Model file for the job. Use its own axes, mm. A direction names the side the tool comes from. Round coordinates to 2 decimals unless told otherwise and drop trailing zeros. Loops run counter-clockwise (first coordinate to the right, second up) from the corner with the lowest first, then second, coordinate; pieces in that order, holes last. Notation, with made-up numbers: M 66.5,35 L 107.5,35 A16 ccw 107.5,61 Z; hole C -13,-7 d8. An arc over 180 degrees is marked long. Use a Markdown table: item, result. Add a question column.
Q1. Cut at B-B (x = 0). Give the cut face in (y, z).
Q2. Cut at A-A (z = 7). Give the cut face in (x, y), plus the area to 3 significant figures.
Q3. Cut at C-C (y = -20). Give the cut face in (x, z).
Q4. Tool access for faces 1 (the face through (-17.062, -15.477, 6.873)), 2 (the face through (19.894, -30.203, 7.194)), 3 (the face through (-6, -20, 2)), 4 (the face through (-19.894, -30.203, 7.194)), 5 (the face through (17.062, -15.477, 6.873)): list every direction of +Z, -Z, +X, -X, +Y, -Y with a clear straight run to the whole face (end or side of a thin tool).
Q5. Probe line 1 (Y direction, x = 0, z = 5.6); line 2 (Y direction, x = 0, z = 1.75); line 3 (X direction, y = -20, z = 1.15). List the from-to ranges inside material, lowest first. Write a range as from..to.
Q6. Pin check, flat tips, straight feed: pin 1 (4 mm diameter, centred on y = -19, z = 4.5, fed in from -X); pin 2 (5 mm diameter, centred on x = 0, y = -20, fed in from +Z); pin 3 (1 mm diameter, centred on x = -5.5, z = 4, fed in from -Y); pin 4 (2 mm diameter, centred on y = -25, z = 4.5, fed in from -X). Stop position of each tip, or through.
Q7. Cut at D-D (x = -16). Give the cut face in (y, z), plus the area to 3 significant figures.
Q8. Mould opens along X. For faces 6 (the face through (3, -17, 4)), 7 (the face through (14.077, -0.376, 3.246)), 8 (the face through (0, 0, 4)), 9 (the face through (-20.23, -30.04, 2.66)) say: +X half, -X half, draft (parallel to the pull), parting line (faces both ways), or undercut.
from build123d import *

# Parameters (mm, degrees)
F0_R     = 3.25
F1_DEPTH = 8.5
F2_R     = 6
F2_R_2   = 3.25
F3_DEPTH = 4
F7_DEPTH = 48.701737703
F8_R     = 1


# Not quite as in the source:
# - a pattern or mirror of a feature is missing from the dataset's text; its kind, count and spacing are read off the source's solid


with BuildPart() as f1:
    # F0 (on Top) → F1 (new body)
    with BuildSketch(Plane.XY):
        with BuildLine():
            Line((21.4749827509, -25.6324591351), (17.0744521737, -4.0031603279))
            ThreePointArc((17.0744521737, -4.0031603279), (15.3383552934, -1.1280367796), (12.1748286506, 0))
            Line((12.1748286506, 0), (0, 0))
            Line((0, 0), (-12.1748286506, 0))
            ThreePointArc((-12.1748286506, 0), (-15.3383552934, -1.1280367796), (-17.0744521737, -4.0031603279))
            Line((-17.0744521737, -4.0031603279), (-21.4749827509, -25.6324591351))
            ThreePointArc((-21.4749827509, -25.6324591351), (-21.1230164973, -28.7074742953), (-19.0284610173, -30.9861659857))
            Line((-19.0284610173, -30.9861659857), (-7.3593053684, -37.5563976295))
            ThreePointArc((-7.3593053684, -37.5563976295), (0, -39.4857960942), (7.3593053684, -37.5563976295))
            Line((7.3593053684, -37.5563976295), (19.0284610173, -30.9861659857))
            ThreePointArc((19.0284610173, -30.9861659857), (21.1230164973, -28.7074742953), (21.4749827509, -25.6324591351))
        make_face()
        with Locations((0, -20)):
            Circle(F0_R, mode=Mode.SUBTRACT)
    extrude(amount=F1_DEPTH)

    # F2 (on face) → F3 (cut)
    with BuildSketch(Plane(origin=(0, 0, 0), x_dir=(1, 0, 0), z_dir=(0, 0, -1))):
        with Locations((0, 20)):
            Circle(F2_R)
        with Locations((0, 20)):
            Circle(F2_R_2, mode=Mode.SUBTRACT)
    extrude(amount=-F3_DEPTH, mode=Mode.SUBTRACT)

    # F6 (on face) → F7 (cut, through all)
    with BuildSketch(Plane(origin=(-8.8517973086, -43.5079737791, 0), x_dir=(-0.9799247046, 0.1993679344, 0), z_dir=(0.1993679344, 0.9799247046, 0))):
        Polygon((15.9335756971, 0), (15.9335756971, 8.5), (13.6335756971, 8.5), (13.6335756971, 5.2), align=None)
    f7 = extrude(amount=F7_DEPTH, mode=Mode.SUBTRACT)

    # F7_copies: F7 across plane
    add(f7.mirror(Plane(origin=(0, 0, 0), x_dir=(0, 0, 1), z_dir=(1, 0, 0))), mode=Mode.SUBTRACT)

    # F8
    f8_edges = [f1.edges().sort_by_distance(p)[0] for p in [
        (-20.060161, -30.214847, 6.85),
        (-13.98162, -0.337865, 6.85),
        (20.060161, -30.214847, 6.85),
        (13.98162, -0.337865, 6.85),
    ]]
    fillet(f8_edges, radius=F8_R)


solid = f1.part
Checked values:
| question | item | result |
|---|---|---|
| 1 | outline | M -39.49,0 L -26,0 L -26,4 L -23.25,4 L -23.25,8.5 L -39.49,8.5 Z; M -16.75,4 L -14,4 L -14,0 L 0,0 L 0,8.5 L -16.75,8.5 Z |
| 2 | outline | M -19.94,-29.64 A1 ccw -19.56,-30.64 A5 ccw -19.03,-30.99 L -7.36,-37.56 A15 ccw 7.36,-37.56 L 19.03,-30.99 A5 ccw 19.56,-30.64 A1 ccw 19.94,-29.64 L 14.1,-0.91 A1 ccw 13.35,-0.14 A5 ccw 12.17,0 L -12.17,0 A5 ccw -13.35,-0.14 A1 ccw -14.1,-0.91 Z; hole C 0,-20 d6.5 |
| 2 | area | 1,220 mm^2 |
| 3 | outline | M -20.33,0 L -6,0 L -6,4 L -3.25,4 L -3.25,8.5 L -17.98,8.5 L -17.98,5.2 Z; M 3.25,4 L 6,4 L 6,0 L 20.33,0 L 17.98,5.2 L 17.98,8.5 L 3.25,8.5 Z |
| 4 | face 1 | +Z, -X, +Y |
| 4 | face 2 | +Z, +X |
| 4 | face 3 | -Z |
| 4 | face 4 | +Z, -X |
| 4 | face 5 | +Z, +X, +Y |
| 5 | line 1 | y = -39.49..-23.25, -16.75..0 |
| 5 | line 2 | y = -39.49..-26, -14..0 |
| 5 | line 3 | x = -19.81..-6, 6..19.81 |
| 6 | pin 1 | stops at x = -19.08 |
| 6 | pin 2 | passes through |
| 6 | pin 3 | stops at y = -38.63 |
| 6 | pin 4 | stops at x = -19.81 |
| 7 | outline | M -32.69,0 L -1.78,0 L -1.78,1.38 L -10.26,5.2 L -10.26,8.5 L -32.69,8.5 Z |
| 7 | area | 219 mm^2 |
| 8 | face 6 | undercut |
| 8 | face 7 | +X half |
| 8 | face 8 | draft |
| 8 | face 9 | -X half |
